For this review, use the dimensioned drawing (mm, ordinates from the lowest corner) and the shaded views. Coordinates: 2 decimals unless noted, no trailing zeros. Loops run counter-clockwise (first coordinate to the right, second up) from the corner with the lowest first, then second, coordinate; pieces in that order, holes last. Notation, with made-up numbers: (85.25, 27) - (140.25, 27) arc R11 ccw to (140.25, 48) - close; hole circle Ø8 at (79, 26.5). An arc over 180 degrees is marked (long way). Answer in a Markdown table with one row per item. Add a question column.
(1) For line 1 along Y through (x, z) = (74, 2.05); line 2 along Y through (x, z) = (104, 1.6); line 3 along X through (y, z) = (50.5, 2.2), list the stretches that pass through material, from the lowest coordinate up.
(2) We need section C-C on y = 52.5. Write out the cut boundary in (x, z).
(3) We need section B-B on x = 104. Write out the cut boundary in (y, z).
(4) We need section A-A on y = 30. Write out the cut boundary in (x, z), plus the area to 3 significant figures.
(5) We need section D-D on z = 2.7. Write out the cut boundary in (x, y), plus the area to 3 significant figures.
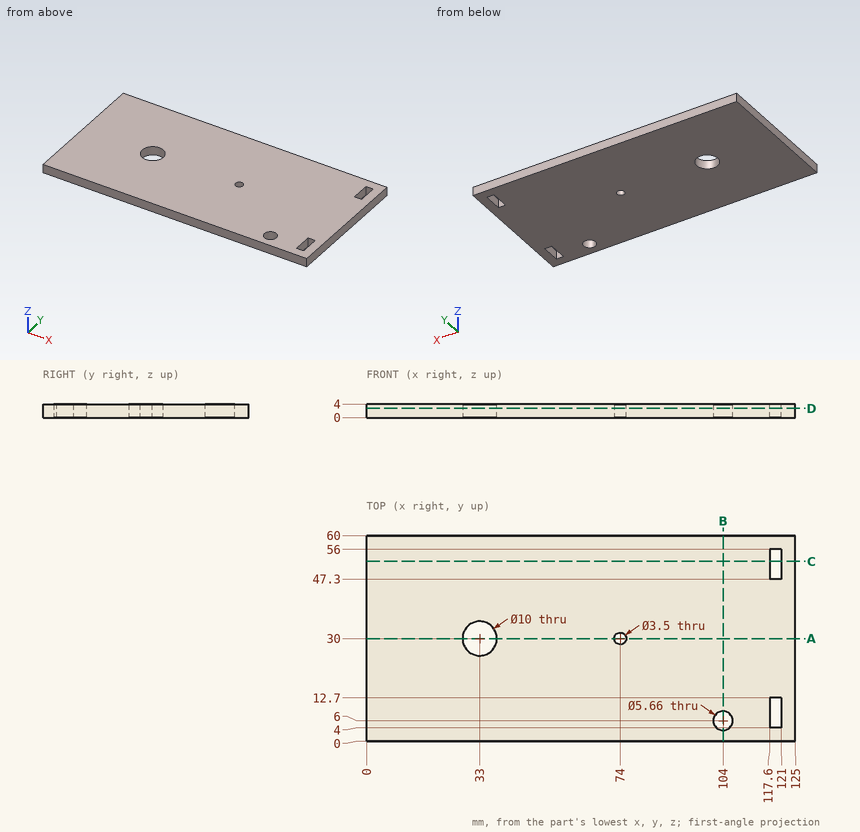
Outcome:
| question | item | result |
|---|---|---|
| 1 | line 1 | 0 to 28.25, 31.75 to 60 |
| 1 | line 2 | 0 to 3.17, 8.83 to 60 |
| 1 | line 3 | 0 to 117.6, 121 to 125 |
| 2 | outline | (0, 0) - (117.6, 0) - (117.6, 4) - (0, 4) - close; (121, 0) - (125, 0) - (125, 4) - (121, 4) - close |
| 3 | outline | (0, 0) - (3.17, 0) - (3.17, 4) - (0, 4) - close; (8.83, 0) - (60, 0) - (60, 4) - (8.83, 4) - close |
| 4 | outline | (0, 0) - (28, 0) - (28, 4) - (0, 4) - close; (38, 0) - (72.25, 0) - (72.25, 4) - (38, 4) - close; (75.75, 0) - (125, 0) - (125, 4) - (75.75, 4) - close |
| 4 | area | 446 mm² |
| 5 | outline | (0, 0) - (125, 0) - (125, 60) - (0, 60) - close; hole circle Ø10 at (33, 30); hole circle Ø3.5 at (74, 30); hole circle Ø5.66 at (104, 6); hole (117.6, 4) - (121, 4) - (121, 12.7) - (117.6, 12.7) - close; hole (117.6, 47.3) - (121, 47.3) - (121, 56) - (117.6, 56) - close |
| 5 | area | 7,330 mm² |
